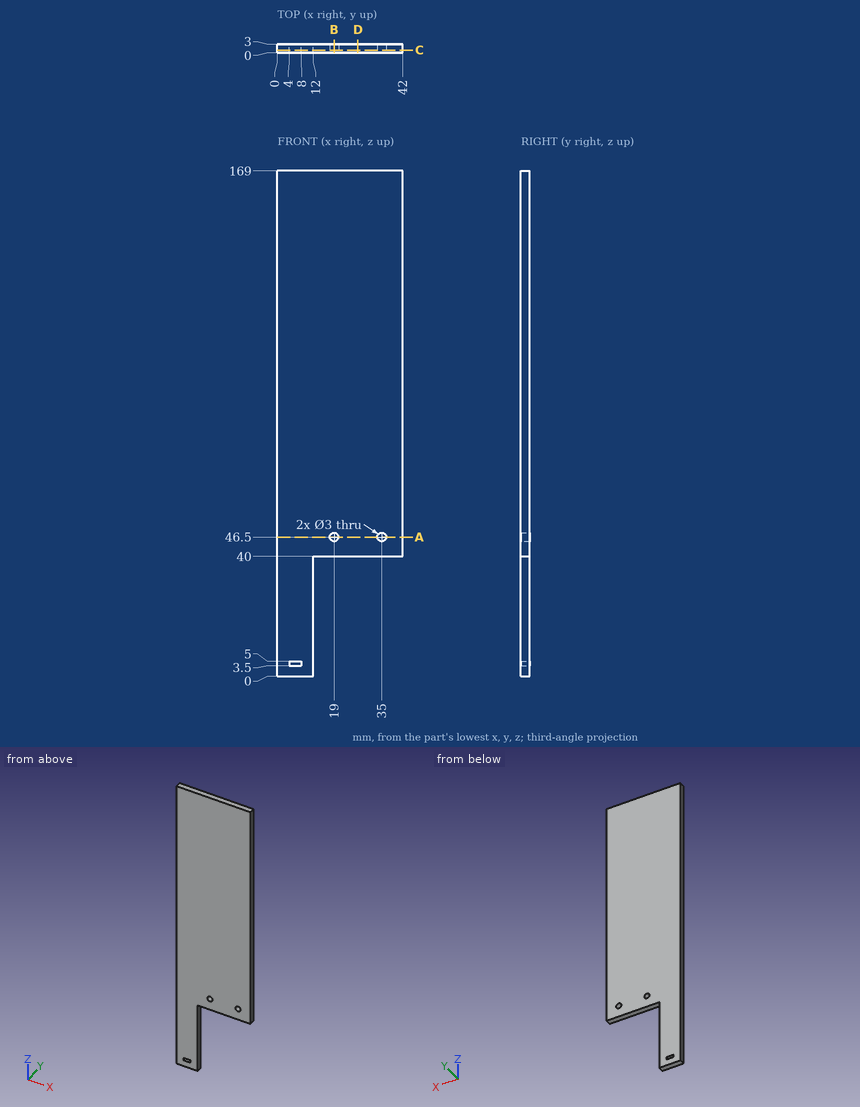
Answer from the drawing. Dimensions are ordinates in mm from the lowest x, y and z of the part. Coordinates: 2 decimals unless noted, no trailing zeros. Write each loop counter-clockwise with the first axis right and the second up, starting at its lowest first coordinate (ties: lowest second). Pieces come first, ordered by that corner, then holes. Notation, with made-up numbers: M 72.25,-30 L 84.25,-30 A10 cw 84.25,-18 Z; hole C 68,1.5 d11. An arc over 180 degrees is marked long. Use one line per item in the form item = value. Start each with the question number.
1. Straight lines are drawn through the part: probe 1 along X at (y, z) = (2.1, 46.5); probe 2 along Z at (x, y) = (5, 2.5); probe 3 along Z at (x, y) = (30, 0.6). For each, find the intervals that lie inside material, in ascending order. Write a range as from..to.
2. The part is cut by section D-D (x = 27). Give the vertices of the cut face in (y, z).
3. The part is cut by section C-C (y = 0.95). Give the vertices of the cut face in (x, z).
4. The part is cut by section B-B (x = 19). Give the vertices of the cut face in (y, z).
5. This flat-tipped pin is pushed along its axis until it touches: P1, Ø0.9, axis at y = 1, z = 12.5, coming from the +X side. Where does it stop, or does it pass through?
6. The part is cut by section A-A (z = 46.5). Give the vertices of the cut face in (x, y).
Evaluation:
q1.probe_1 = 0..17.5, 20.5..33.5, 36.5..42
q1.probe_2 = 0..3.5, 5..169
q1.probe_3 = 40..169
q2.outline = M 0,40 L 3,40 L 3,169 L 0,169 Z
q3.outline = M 0,0 L 12,0 L 12,40 L 42,40 L 42,169 L 0,169 Z; hole M 4,3.5 L 8,3.5 L 8,5 L 4,5 Z; hole C 19,46.5 d3; hole C 35,46.5 d3
q4.outline = M 0,40 L 3,40 L 3,45 L 0,45 Z; M 0,48 L 3,48 L 3,169 L 0,169 Z
q5.P1 = 12
q6.outline = M 0,0 L 17.5,0 L 17.5,3 L 0,3 Z; M 20.5,0 L 33.5,0 L 33.5,3 L 20.5,3 Z; M 36.5,0 L 42,0 L 42,3 L 36.5,3 Z
